Work out the finished part from the listing and answer in its coordinate system (mm). A direction names the side the tool comes from. Give positions to 0.01 mm unless a question says otherwise; leave off trailing zeros. Order: outer loops, then holes, each group sorted by start corner. A loop starts at its lowest first (then second) coordinate and runs counter-clockwise, first axis right, second up. Notation, with made-up numbers: (-19, -15) - (3, -15) arc R25 cw to (3, 13) - close; hole circle Ø8 at (-22, -6). An arc over 180 degrees is marked (long way). Put each result on its own line as item: value.
```python
from build123d import *

# Parameters (mm, degrees)
SKETCH2_W           = 19.5
SKETCH2_H           = 10
SKETCH2_R           = 1.5
BOSS_EXTRUDE1_DEPTH = 1.27
SKETCH3_W           = 19.05
SKETCH3_H           = 10
BOSS_EXTRUDE2_DEPTH = 2.54
SKETCH4_R           = 1.75
CUT_EXTRUDE1_DEPTH  = 26.075286638


with BuildPart() as part:
    # Sketch2 → Boss-Extrude1 (new, symmetric)
    with BuildSketch(Plane.XY):
        Rectangle(SKETCH2_W, SKETCH2_H)
        with Locations((-4.75, -2.5)):
            Circle(SKETCH2_R, mode=Mode.SUBTRACT)
        with Locations((4.75, -2.5)):
            Circle(SKETCH2_R, mode=Mode.SUBTRACT)
    extrude(amount=BOSS_EXTRUDE1_DEPTH, both=True)

    # Sketch3 → Boss-Extrude2 (add)
    with BuildSketch(Plane.ZY.offset(9.75)):
        with Locations((8.255, 0)):
            Rectangle(SKETCH3_W, SKETCH3_H)
    extrude(amount=-BOSS_EXTRUDE2_DEPTH)

    # Sketch4 → Cut-Extrude1 (cut, through all)
    with BuildSketch(Plane(origin=(-7.21, 0, 0), x_dir=(0, 0, -1), z_dir=(1, 0, 0))):
        with Locations((-5.715, 0)):
            Circle(SKETCH4_R)
        with Locations((-13.335, 0)):
            Circle(SKETCH4_R)
    extrude(amount=-CUT_EXTRUDE1_DEPTH, mode=Mode.SUBTRACT)


solid = part.part
```
(1) A tool of negligible diameter and unlimited length cuts with its end or side. For faces 5 (the face through (-5.86, -1.49, -0.02)), 6 (the face through (-7.21, 0, 9)), from which of +Z, -Z, +X, -X, +Y, -Y can it reach the whole face along a straight path? Write none if from no direction.
Geometry check:
face 5: +Z, -Z
face 6: +Z, +X, +Y, -Y
(2) Section D-D, the plane y = -2.5 is taken. Write down the section's boundary in (x, z), then the cut area to 3 significant figures.
Geometry check:
outline: (-9.75, -1.27) - (-6.25, -1.27) - (-6.25, 1.27) - (-7.21, 1.27) - (-7.21, 17.78) - (-9.75, 17.78) - close; (-3.25, -1.27) - (3.25, -1.27) - (3.25, 1.27) - (-3.25, 1.27) - close; (6.25, -1.27) - (9.75, -1.27) - (9.75, 1.27) - (6.25, 1.27) - close
area: 76.2 mm²
(3) Section C-C, the plane z = 4.75 is taken. Write down the section's boundary in (x, y).
Geometry check:
outline: (-9.75, -5) - (-7.21, -5) - (-7.21, -1.46) - (-9.75, -1.46) - close; (-9.75, 1.46) - (-7.21, 1.46) - (-7.21, 5) - (-9.75, 5) - close
(4) Section A-A, the plane x = 4.75 is taken. Write down the section's boundary in (y, z).
Geometry check:
outline: (-5, -1.27) - (-4, -1.27) - (-4, 1.27) - (-5, 1.27) - close; (-1, -1.27) - (5, -1.27) - (5, 1.27) - (-1, 1.27) - close
(5) Section B-B, the plane y = 0 is taken. Write down the section's boundary in (x, z) (3 decimals), then the cut area to 3 significant figures.
Geometry check:
outline: (-9.75, -1.27) - (9.75, -1.27) - (9.75, 1.27) - (-7.21, 1.27) - (-7.21, 3.965) - (-9.75, 3.965) - close; (-9.75, 7.465) - (-7.21, 7.465) - (-7.21, 11.585) - (-9.75, 11.585) - close; (-9.75, 15.085) - (-7.21, 15.085) - (-7.21, 17.78) - (-9.75, 17.78) - close
area: 73.7 mm²
(6) Determine the mould class of faces 1 (the face through (-8.462, 0.526, 11.666)), 2 (the face through (1, 0, 1.27)), 3 (the face through (0, 0, -1.27)), 4 (the face through (5.556, -1.235, -0.018)) for opening direction Z: pulls with the +Z half, pulls with the -Z half, needs draft (parallel to the pull), parting line crosses it, or undercut.
Geometry check:
face 1: undercut
face 2: pulls with the +Z half
face 3: pulls with the -Z half
face 4: needs draft
(7) Given pin 1 (5 mm diameter, centred on y = -0.5, z = 12, fed in from +X); pin 2 (5 mm diameter, centred on x = 4.5, y = -2.5, fed in from +Z), each flat-ended and moving along its own axis, determine where each tip first touches the part or whether it passes through.
Geometry check:
pin 1: stops at x = -7.21
pin 2: stops at z = 1.27
(8) Straight lines are drawn through the part: line 1 (Y direction, x = 4.75, z = -0.05); line 2 (Z direction, x = -7.5, y = 1); line 3 (Z direction, x = -5, y = 1). For each, find the intervals that lie inside material, in ascending order.
Geometry check:
line 1: y = -5 to -4, -1 to 5
line 2: z = -1.27 to 4.28, 7.15 to 11.9, 14.77 to 17.78
line 3: z = -1.27 to 1.27
